Autodesk Inventor part; units mm, degrees
ref_plane "YZ Plane" through (0, 0, 0) normal (1, 0, 0) x (0, 1, 0)
ref_plane "XZ Plane" through (0, 0, 0) normal (0, 1, 0) x (-1, 0, 0)
ref_plane "XY Plane" through (0, 0, 0) normal (0, 0, 1) x (1, 0, 0)
sketch "Szkic1" plane through (0, 0, 0) normal (0, 1, 0) x (-1, 0, 0)
  line L0 (0, 0) -> (45, 0)
  line L1 (45, 0) -> (45, -30)
  line L2 (45, -30) -> (0, -30)
  line L3 (0, -30) -> (0, 0)
  line L4 (45, 0) -> (45, 2)
  line L5 (45, 2) -> (47, 2)
  line L6 (0, -30) -> (0, -32)
  line L7 (0, -32) -> (-2, -32)
  line L8 (-2, -32) -> (47, -32)
  line L9 (47, -32) -> (47, 2)
  line L10 (47, 2) -> (-2, 2)
  line L11 (-2, 2) -> (-2, -32)
  line L12 (47, 2) -> (47, 17)
  line L13 (-2, 2) -> (-2, 17)
  line L14 (-2, 17) -> (47, 17)
  line L15 (-2, 17) -> (-2, 15)
  line L16 (-2, 15) -> (47, 15)
  line L17 (47, 17) -> (47, 14.5669)
  line L18 (0, 2) -> (0, 15)
  line L19 (45, 2) -> (45, 15)
  line L20 (0, 0) -> (0, 2)
  line L21 (45, 0) -> (45, 2)
  dimension "d0" = 45
  dimension "d1" = 30
  dimension "d2" = 2
  dimension "d3" = 2
  dimension "d4" = 2
  dimension "d5" = 2
  dimension "d40" = 15
  dimension "d41" = 15
  dimension "d42" = 2
extrude "Wyciągnięcie proste1" add sketch "Szkic1" along normal blind 20 contours L3 L6 L7 L11 L10 L20 | L4 L5 L9 L8 L6 L2 L1 | L10 L13 L16 L18 | L19 L16 L12 L5 | L16 L13 L14 L12
sketch "Szkic2" plane through (0, 0, 0) normal (0, -1, 0) x (1, 0, 0)
  line L0 (-47, 2) -> (2, 2)
  line L1 (-47, -32) -> (-47, 17)
  line L2 (2, 2) -> (-47, 2)
  line L3 (-47, 2) -> (-47, -32)
  line L4 (-47, -32) -> (2, -32)
  line L5 (2, -32) -> (2, 2)
  point P0 (0, 0)
extrude "Wyciągnięcie proste2" add sketch "Szkic2" against normal blind 2
sketch "Szkic3" plane through (2, 0, -32) normal (0, 0, -1) x (-1, 0, 0)
  line L0 (40, 2) -> (15, 2)
  line L1 (15, 2) -> (15, 14)
  line L2 (15, 14) -> (40, 14)
  line L3 (40, 14) -> (40, 2)
  line L4 (40, 14) -> (38, 14)
  line L5 (38, 14) -> (38, 2)
  line L6 (38, 2) -> (40, 2)
  line L7 (40, 2) -> (40, 14)
  point P0 (2, 0)
  dimension "d10" = 25
  dimension "d11" = 12
  dimension "d30" = 2
extrude "Wyciągnięcie proste3" cut sketch "Szkic3" against normal blind 4.5 contours L0 L1 L2 L5
sketch "Szkic4" plane through (0, 20, 0) normal (0, 0, -1) x (-1, 0, 0)
  line L0 (38, -6) -> (38, -18)
  line L1 (38, -12) -> (28, -12)
  line L2 (28, -12) -> (30.5, -12)
  circle A0 centre (30.5, -12) radius 4.5
  line L3 (13, -6) -> (36, -6)
  line L4 (24.5, -6) -> (24.5, -18)
  line L5 (0, -18) -> (45, -18)
  line L6 (11, -12) -> (21, -12)
  circle A1 centre (18.5, -12) radius 4.5
  point P0 (0, -20)
  dimension "d14" = 10
  dimension "d15" = 2.5
  dimension "d16" = 9
extrude "Wyciągnięcie proste4" [suppressed]
sketch "Szkic5" plane through (0, 20, 0) normal (0, 1, 0) x (1, 0, 0)
  line L0 (0, 30) -> (0, 0)
  line L1 (2, -17) -> (2, 32)
  line L2 (0, 9.9645) -> (2, 9.9645)
  line L3 (2, 9.9645) -> (2, 19.9645)
  line L4 (2, 19.9645) -> (0, 19.9645)
  line L5 (0, 19.9645) -> (0, 9.9645)
  point P0 (2, -2)
  dimension "d19" = 10
extrude "Wyciągnięcie proste5" cut sketch "Szkic5" against normal blind 18
sketch "Szkic6" plane through (-47, 0, 2) normal (0, 0, 1) x (1, 0, 0)
  circle A0 centre (28.5, 8) radius 4.5
  line L0 (28.5, 8) -> (28.5, -2)
  circle A1 centre (28.5, 8) radius 3.5
  circle A2 centre (28.5, 8) radius 4.5
  point P0 (47, 0)
  dimension "d22" = 10
  dimension "d27" = 7
sketch "Szkic7" plane through (0, 0, 0) normal (0, -1, 0) x (1, 0, 0)
  line L0 (2, 17) -> (2, -32)
  line L1 (-47, -32) -> (2, -32)
  line L2 (2, -32) -> (2, 2)
  line L3 (2, 2) -> (-47, 2)
  line L4 (-47, 2) -> (-47, -32)
  line L5 (-47, 17) -> (2, 17)
  line L6 (-47, 0) -> (2, 0)
  line L7 (2, 0) -> (2, 17)
  line L8 (2, 17) -> (-47, 17)
  line L9 (-47, 17) -> (-47, 0)
  point P0 (0, 0)
extrude "Wyciągnięcie proste6" add sketch "Szkic7" along normal blind 3
sketch "Szkic8" plane through (0, 2, 0) normal (0, 1, 0) x (1, 0, 0)
  line L0 (-45, -2) -> (-45, 30)
  line L1 (0, 9.9645) -> (0, 0)
  line L2 (-45, 0) -> (0, 0)
  line L3 (0, 0) -> (0, 9.9645)
  line L4 (0, 9.9645) -> (-45, 9.9645)
  line L5 (-45, 9.9645) -> (-45, 0)
extrude "Wyciągnięcie proste7" cut sketch "Szkic8" against normal blind 4
extrude "Wyciągnięcie proste8" [suppressed]
sketch "Szkic9" plane through (2, 20, -32) normal (0, 0, -1) x (-1, 0, 0)
  line L0 (15, -6) -> (15, -18)
  line L1 (15, -12) -> (20.5, -12)
  circle A0 centre (20.5, -12) radius 3.5
  line L2 (0, -20) -> (0, -23)
  line L3 (0, -11.5) -> (29.45, -11.5)
  line L4 (0, -11.5) -> (23.29, -11.5)
  line L5 (23.29, -11.5) -> (20.94, -11.5)
  line L6 (20.94, -11.5) -> (20.94, -12)
  circle A1 centre (20.94, -12) radius 3.5
  point P0 (2, -20)
  point P1 (0, 0)
  dimension "d31" = 5.5
  dimension "d32" = 7
  dimension "d35" = 29.45
  dimension "d36" = 23.29
  dimension "d37" = 2.35
  dimension "d38" = 7
extrude "Wyciągnięcie proste9" cut sketch "Szkic9" against normal blind 47.25 contours A1 L3 A0 | A0 L3 A1 | L3 A0 A1 | A0 L3 A1 picked at (24.181, -11.2212) picked at (22.5407, -11.0097) picked at (22.6367, -12.1539) picked at (24.2617, -12.2698)
sketch "Szkic11" plane through (0, -2, 0) normal (0, 1, 0) x (1, 0, 0)
  line L0 (0, -15) -> (-45, -15)
  line L1 (-45, 9.9645) -> (-45, 30)
  line L2 (0, -15) -> (-45, -15)
  line L3 (-45, -15) -> (-45, 9.9645)
  line L4 (-45, 9.9645) -> (0, 9.9645)
  line L5 (0, 9.9645) -> (0, -15)
  point P0 (0, 0)
extrude "Wyciągnięcie proste10" cut sketch "Szkic11" along normal blind 43.5
sketch "Szkic12" plane through (-18.94, 8, 15.25) normal (0, 0, -1) x (-1, 0, 0)
  point P0 (-18.94, -8)
sketch "Szkic14" plane through (2, 20, -32) normal (0, 0, -1) x (-1, 0, 0)
  line L0 (0, -23) -> (0, 0)
  line L1 (0, -11.5) -> (29.51, -11.5)
  line L2 (0, -11.5) -> (29.51, -11.5) construction
  line L3 (29.51, -11.5) -> (18.2, -11.5)
  line L4 (18.2, -11.5) -> (20.515, -11.5)
  circle A0 centre (20.515, -11.5) radius 3.25
  point P0 (2, -20)
  dimension "d47" = 29.51
  dimension "d48" = 0
  dimension "d49" = 11.31
  dimension "d50" = 2.315
  dimension "d51" = 6.5
extrude "Wyciągnięcie proste11" cut sketch "Szkic14" against normal through all
sketch "Szkic15" plane through (0, 20, 15) normal (0, 0, -1) x (-1, 0, 0)
  arc A0 (20.2611, -8.7589) -> (15.5284, -12.7817) centre (18.515, -11.5) ccw
  circle A1 centre (18.515, -11.5) radius 3.25
  arc A2 (15.5284, -12.7817) -> (20.2611, -8.7589) centre (18.94, -12) ccw
  arc A3 (15.5284, -12.7817) -> (20.2611, -8.7589) centre (18.94, -12) ccw
  point P0 (0, -20)
  point P1 (15.5284, -12.7817)
extrude "Wyciągnięcie proste12" add sketch "Szkic15" against normal blind 2 contours A2 A1
sketch "Szkic16" plane through (2, 2, -9.9645) normal (1, 0, 0) x (0, 0, -1)
  line L0 (22.0355, 18) -> (22.0355, -5)
  line L1 (22.0355, -5) -> (-26.9645, -5)
  line L2 (22.0355, 18) -> (18.0355, 18)
  line L3 (18.0355, 18) -> (18.0355, -5)
  line L4 (18.0355, -5) -> (22.0355, -5)
  line L5 (22.0355, -5) -> (22.0355, 18)
  line L6 (-26.9645, 18) -> (-22.9645, 18)
  line L7 (-22.9645, 18) -> (-22.9645, -5)
  line L8 (-22.9645, -5) -> (-26.9645, -5)
  line L9 (-26.9645, -5) -> (-26.9645, 18)
  point P0 (-9.9645, -2)
  point P1 (-22.9645, -5)
  dimension "d56" = 4
  dimension "d57" = 4
sketch "Szkic17" plane through (2, 20, -32) normal (0, 0, -1) x (-1, 0, 0)
  circle A0 centre (20.515, -11.5) radius 3.25
  line L0 (20.515, -11.5) -> (-79.485, -11.5)
  point P0 (2, -20)
  dimension "d58" = 100
extrude "Wyciągnięcie proste13" add sketch "Szkic16" along normal blind 79.5
sketch "Szkic18" plane through (-47, -3, -32) normal (0, 0, -1) x (-1, 0, 0)
  line L0 (-128.5, 0) -> (-128.5, 23)
  circle A0 centre (-128.5, 11.5) radius 2.85
  line L1 (-128.5, 11.5) -> (-118.5, 11.5)
  line L2 (-118.5, 11.5) -> (-118.5, 5)
  line L3 (-118.5, 5) -> (-146.5, 5)
  line L4 (-146.5, 18) -> (-118.5, 18)
  line L5 (-118.5, 18) -> (-118.5, 11.5)
  line L6 (-128.5, 18) -> (-128.5, 5)
  line L7 (-138.5, 11.5) -> (-138.5, 5)
  line L8 (-138.5, 5) -> (-110.5, 5)
  line L9 (-110.5, 5) -> (-110.5, 18)
  line L10 (-110.5, 18) -> (-138.5, 18)
  line L11 (-138.5, 18) -> (-138.5, 11.5)
  point P0 (-47, 3)
  dimension "d61" = 5.7
  dimension "d62" = 10
  dimension "d63" = 6.5
  dimension "d64" = 28
  dimension "d65" = 13
sketch "Szkic19" plane through (81.5, 2, -9.9645) normal (1, 0, 0) x (0, 0, -1)
  line L0 (-26.9645, -5) -> (-26.9645, 18)
  line L1 (-26.9645, -5) -> (22.0355, -5)
  line L2 (-26.9645, 18) -> (-22.9645, 18)
  line L3 (-22.9645, 18) -> (-22.9645, -5)
  line L4 (-22.9645, -5) -> (-26.9645, -5)
  line L5 (-26.9645, -5) -> (-26.9645, 18)
  line L6 (22.0355, 18) -> (18.0355, 18)
  line L7 (18.0355, 18) -> (18.0355, -5)
  line L8 (18.0355, -5) -> (22.0355, -5)
  line L9 (22.0355, -5) -> (22.0355, 18)
  point P0 (-9.9645, -2)
  dimension "d66" = 4
  dimension "d67" = 4
extrude "Wyciągnięcie proste14" add sketch "Szkic19" along normal blind 10
extrude "Wyciągnięcie proste15" cut sketch "Szkic18" against normal blind 11.5 contours A0 L0 | L0 L1 A0 | L0 A0 L1
sketch "Szkic20" plane through (-47, -3, 17) normal (0, 0, 1) x (1, 0, 0)
  point P0 (47, 3)
sketch "Szkic21" plane through (-47, -3, 17) normal (0, 0, 1) x (1, 0, 0)
  circle A0 centre (128.5, 11.5) radius 2.85
  circle A1 centre (128.5, 11.5) radius 2.95
  point P0 (47, 3)
  dimension "d72" = 5.9
extrude "Wyciągnięcie proste16" cut sketch "Szkic21" against normal blind 25.25 contours A0
fillet "Zaokrąglenie1" radius 11.5 4 edges at (91.5, 20, -30) (91.5, -3, -30) (91.5, 20, 15) (91.5, -3, 15)
ref_plane "Płaszczyzna konstrukcyjna2" through (91.5, 8.5, 16.5) normal (0, 0, -1) x (-1, 0, 0)
ref_plane "Płaszczyzna konstrukcyjna1" through (91.5, 8.5, 17) normal (0, 0, -1) x (-1, 0, 0)
sketch "Szkic22" plane through (91.5, 8.5, 16.5) normal (0, 0, -1) x (-1, 0, 0)
  circle A0 centre (10, 0) radius 2.85
  circle A1 centre (10, 0) radius 1.5
  circle A2 centre (10, 0) radius 2.85
  point P0 (91.5, -8.5)
  dimension "d77" = 3
extrude "Wyciągnięcie proste17" add sketch "Szkic22" along normal blind 0.25
sketch "Szkic23" plane through (0, 20, 0) normal (0, 1, 0) x (1, 0, 0)
  point P0 (0, 0)
properties part number "servo_box"
Build history of the part. All positions in model axes, mm. A direction names the side the tool comes from. Round coordinates to 2 decimals unless told otherwise and drop trailing zeros. Write each loop counter-clockwise with the first axis right and the second up, starting at its lowest first coordinate (ties: lowest second). Pieces come first, ordered by that corner, then holes.
1) Pin check, flat tips, straight feed: pin 1 (12 mm diameter, centred on x = 16, z = 6, fed in from +Y); pin 2 (10 mm diameter, centred on y = 8.5, z = -7.5, fed in from +X); pin 3 (3.5 mm diameter, centred on x = 81.5, y = 8.5, fed in from +Z). Stop position of each tip, or through.
2) Band-saw the part on A-A, the plane x = 70.5. List the corners of the cut face in (y, z).
3) 3-axis set-ups, long thin cutter, end or side, ignore diameter. For faces 1 (the flat face through (0, 11, -25)), 2 (the cylindrical face through (83.032, 10.903, 14.648)), 3 (the flat face through (80, 7, 16.5)), 4 (the flat face through (2, 8, -7)): which of +Z, -Z, +X, -X, +Y, -Y reach the whole face in a straight line?
4) Band-saw the part on D-D, the plane x = -29.5. List the corners of the cut face in (y, z).
5) Drill centre lines: probe 1 along X at (y, z) = (8.5, 16.6) (3 decimals); probe 2 along Z at (x, y) = (49, 17); probe 3 along X at (y, z) = (12.75, 10). Where is each one in solid material? Low to high.
6) Mould opens along Z. For faces 5 (the flat face through (21, 8, -32)), 6 (the cylindrical face through (-21.615, 9.476, 15.986)), 7 (the flat face through (-22, 2, -21)) say: +Z half, -Z half, draft (parallel to the pull), parting line (faces both ways), or undercut.
7) Band-saw the part on B-B, the plane z = -25. List the corners of the cut face in (x, y).
8) Band-saw the part on C-C, the plane y = 8.5. Give the number of separate pieces and of enclosed holes in the cut face, and give its area (3 significant figures).
Ans:
1. pin 1: passes through
1. pin 2: stops at x = 2
1. pin 3: stops at z = 16.5
2. outline: (-3, -32) - (20, -32) - (20, -28) - (-3, -28) - close; (-3, 13) - (20, 13) - (20, 17) - (-3, 17) - close
3. face 1: +Y
3. face 2: -Z
3. face 3: +Z
3. face 4: +X, +Y, -Y
4. outline: (-3, -32) - (2, -32) - (2, -9.96) - (-2, -9.96) - (-2, 15) - (20, 15) - (20, 17) - (-3, 17) - close; (14, -32) - (20, -32) - (20, -30) - (14, -30) - close
5. probe 1: x = -47 to -21.765, -15.265 to 78.65, 84.35 to 91.5
5. probe 2: z = -32 to -28, 13 to 17
5. probe 3: x = -47 to -45, 0 to 2
6. face 5: -Z half
6. face 6: draft
6. face 7: undercut
7. outline: (-47, -3) - (2, -3) - (2, 20) - (0, 20) - (0, 2) - (-45, 2) - (-45, 20) - (-47, 20) - close
8. separate pieces: 5
8. enclosed holes: 0
8. area: 968 mm2
